Geometry: final body of the model. Coordinates: model frame, mm. A direction names the side the tool comes from. Round coordinates to 2 decimals unless told otherwise and drop trailing zeros. Loops run counter-clockwise (first coordinate to the right, second up) from the corner with the lowest first, then second, coordinate; pieces in that order, holes last. Notation, with made-up numbers: (3.5, 75.5) - (35.5, 75.5) arc R21 ccw to (35.5, 113.5) - close; hole circle Ø7 at (21.5, -1.5). An arc over 180 degrees is marked (long way). Use CSV: the item, a comma, the result in double quotes.
from build123d import *

# Parameters (mm, degrees)
SKETCH1_W            = 76.2
SKETCH1_H            = 76.2
BOSS_EXTRUDE1_DEPTH  = 1.5875
SKETCH3_W            = 6.35
SKETCH3_H            = 3.175
SKETCH3_W_2          = 3.175
SKETCH3_H_2          = 6.35
BOSS_EXTRUDE2_DEPTH  = 12.7
SKETCH4_W            = 6.35
SKETCH4_H            = 14.2875
BOSS_EXTRUDE3_DEPTH  = 7.62
SKETCH5_W            = 14.2875
SKETCH5_H            = 6.35
BOSS_EXTRUDE4_DEPTH  = 7.62
SKETCH6_W            = 14.2875
SKETCH6_H            = 6.35
BOSS_EXTRUDE5_DEPTH  = 7.62
SKETCH7_R            = 1.984375
CUT_EXTRUDE2_DEPTH   = 67.217591743
BOSS_EXTRUDE6_DEPTH  = 76.2
CUT_EXTRUDE3_REACH   = 89.333
SKETCH9_W            = 63.5
SKETCH9_H            = 12.7
BOSS_EXTRUDE7_DEPTH  = 6.35
BOSS_EXTRUDE8_DEPTH  = 6.35
SKETCH12_W           = 7.62
SKETCH12_H           = 12.7
SKETCH12_R           = 1.984375
CUT_EXTRUDE4_DEPTH   = 30.48
SKETCH13_W           = 6.35
SKETCH13_H           = 7.62
CUT_EXTRUDE5_DEPTH   = 30.48
SKETCH15_W           = 6.35
SKETCH15_H           = 12.7
CUT_EXTRUDE6_DEPTH   = 30.48
BOSS_EXTRUDE9_DEPTH  = 14.2875
SKETCH17_R           = 2.5
CUT_EXTRUDE7_DEPTH   = 24.9555
SKETCH18_R           = 2.5
CUT_EXTRUDE8_DEPTH   = 11.43
BOSS_EXTRUDE10_DEPTH = 3.556
SKETCH20_W           = 16
SKETCH20_H           = 16
SKETCH20_R           = 2.5
BOSS_EXTRUDE11_DEPTH = 14.2875
SKETCH21_R           = 2.5
CUT_EXTRUDE9_DEPTH   = 31.0515
SKETCH22_R           = 2.5
CUT_EXTRUDE10_DEPTH  = 10.16
SKETCH23_W           = 23.556
SKETCH23_H           = 14.2875
BOSS_EXTRUDE12_DEPTH = 1.27
SKETCH24_W           = 6.35
SKETCH24_H           = 7.62
CUT_EXTRUDE11_DEPTH  = 30.988
SKETCH25_W           = 7.62
SKETCH25_H           = 12.7
CUT_EXTRUDE12_DEPTH  = 30.988
SKETCH26_W           = 12.7
SKETCH26_H           = 12.7
BOSS_EXTRUDE13_DEPTH = 12.192
SKETCH28_W           = 12.7
SKETCH28_H           = 12.7
BOSS_EXTRUDE15_DEPTH = 12.2555
SKETCH29_W           = 12.7
SKETCH29_H           = 12.367297847
BOSS_EXTRUDE16_DEPTH = 8.9535
SKETCH30_W           = 6.317197846
SKETCH30_H           = 6.27
CUT_EXTRUDE13_DEPTH  = 32.8295
SKETCH27_W           = 10
SKETCH27_H           = 10
BOSS_EXTRUDE17_DEPTH = 14.2875


with BuildPart() as part:
    # Sketch1 → Boss-Extrude1 (new body)
    with BuildSketch(Plane.XY):
        Rectangle(SKETCH1_W, SKETCH1_H)
    extrude(amount=BOSS_EXTRUDE1_DEPTH)

    # Sketch3 → Boss-Extrude2 (add)
    with BuildSketch(Plane.XY.offset(1.5875)):
        with Locations((-34.925, 36.5125)):
            Rectangle(SKETCH3_W, SKETCH3_H)
        with Locations((34.925, 36.5125)):
            Rectangle(SKETCH3_W, SKETCH3_H)
        with Locations((-36.5125, -34.925)):
            Rectangle(SKETCH3_W_2, SKETCH3_H_2)
        with Locations((36.5125, -34.925)):
            Rectangle(SKETCH3_W_2, SKETCH3_H_2)
    extrude(amount=BOSS_EXTRUDE2_DEPTH)

    # Sketch4 → Boss-Extrude3 (add)
    with BuildSketch(Plane(origin=(0, 38.1, 0), x_dir=(1, 0, 0), z_dir=(0, 1, 0))):
        with Locations((-34.925, -7.14375)):
            Rectangle(SKETCH4_W, SKETCH4_H)
        with Locations((34.925, -7.14375)):
            Rectangle(SKETCH4_W, SKETCH4_H)
    extrude(amount=BOSS_EXTRUDE3_DEPTH)

    # Sketch5 → Boss-Extrude4 (add)
    with BuildSketch(Plane(origin=(38.1, 0, 0), x_dir=(0, 0, -1), z_dir=(1, 0, 0))):
        with Locations((-7.14375, -34.925)):
            Rectangle(SKETCH5_W, SKETCH5_H)
    extrude(amount=BOSS_EXTRUDE4_DEPTH)

    # Sketch6 → Boss-Extrude5 (add)
    with BuildSketch(Plane.ZY.offset(38.1)):
        with Locations((7.14375, -34.925)):
            Rectangle(SKETCH6_W, SKETCH6_H)
    extrude(amount=BOSS_EXTRUDE5_DEPTH)

    # Sketch7 → Cut-Extrude2 (cut, through all)
    with BuildSketch(Plane(origin=(0, 0, 0), x_dir=(-1, 0, 0), z_dir=(0, 0, -1))):
        with Locations((-34.925, 41.39168957)):
            Circle(SKETCH7_R)
        with Locations((34.925, 41.39168957)):
            Circle(SKETCH7_R)
        with Locations((-41.275, -34.925)):
            Circle(SKETCH7_R)
        with Locations((41.275, -34.925)):
            Circle(SKETCH7_R)
    extrude(amount=-CUT_EXTRUDE2_DEPTH, mode=Mode.SUBTRACT)

    # Sketch8 → Boss-Extrude6 (add)
    with BuildSketch(Plane.ZY.offset(38.1)):
        Polygon((1.5875, 25.732702153), (14.2875, 34.925), (1.5875, 34.925), align=None)
    extrude(amount=-BOSS_EXTRUDE6_DEPTH)

    # Sketch9 → Cut-Extrude3 (cut, up to next)
    with BuildSketch(Plane(origin=(0, 34.925, 0), x_dir=(1, 0, 0), z_dir=(0, 1, 0)), mode=Mode.PRIVATE) as cut_extrude3_sk1:
        with Locations((0, -7.9375)):
            Rectangle(SKETCH9_W, SKETCH9_H)
    cut_extrude3_tool1 = extrude(cut_extrude3_sk1.sketch, amount=-CUT_EXTRUDE3_REACH, mode=Mode.PRIVATE) & part.part
    add(cut_extrude3_tool1.solids().sort_by_distance((0, 34.925, 7.9375))[0], mode=Mode.SUBTRACT)

    # Sketch10 → Boss-Extrude7 (add)
    with BuildSketch(Plane.XZ.offset(38.1)):
        Polygon((-26.257396371, 1.5875), (-34.925, 14.2875), (-34.925, 1.5875), align=None)
        Polygon((34.925, 14.2875), (26.257396371, 1.5875), (34.925, 1.5875), align=None)
    extrude(amount=-BOSS_EXTRUDE7_DEPTH)

    # Sketch11 → Boss-Extrude8 (add)
    with BuildSketch(Plane.XZ.offset(38.1)):
        Polygon((-45.72, 14.2875), (-45.72, 0), (45.72, 0), (45.72, 14.2875), (34.925, 14.2875), (26.257396371, 1.5875), (-26.257396371, 1.5875), (-34.925, 14.2875), align=None)
    extrude(amount=BOSS_EXTRUDE8_DEPTH)

    # Sketch12 → Cut-Extrude4 (cut)
    with BuildSketch(Plane(origin=(0, 0, 0), x_dir=(-1, 0, 0), z_dir=(0, 0, -1))):
        with Locations((-41.91, -38.1)):
            Rectangle(SKETCH12_W, SKETCH12_H)
        with Locations((-41.275, -34.925)):
            Circle(SKETCH12_R, mode=Mode.SUBTRACT)
    extrude(amount=-CUT_EXTRUDE4_DEPTH, mode=Mode.SUBTRACT)

    # Sketch13 → Cut-Extrude5 (cut)
    with BuildSketch(Plane(origin=(0, 0, 0), x_dir=(-1, 0, 0), z_dir=(0, 0, -1))):
        with Locations((-34.925, 41.91)):
            Rectangle(SKETCH13_W, SKETCH13_H)
    extrude(amount=-CUT_EXTRUDE5_DEPTH, mode=Mode.SUBTRACT)

    # Sketch15 → Cut-Extrude6 (cut)
    with BuildSketch(Plane(origin=(0, 38.1, 0), x_dir=(1, 0, 0), z_dir=(0, 1, 0))):
        with Locations((34.925, -7.9375)):
            Rectangle(SKETCH15_W, SKETCH15_H)
    extrude(amount=-CUT_EXTRUDE6_DEPTH, mode=Mode.SUBTRACT)

    # Sketch16 → Boss-Extrude9 (add)
    with BuildSketch(Plane(origin=(0, 0, 0), x_dir=(-1, 0, 0), z_dir=(0, 0, -1))):
        Polygon((-38.1, 38.1), (-38.1, 43.1), (-18.1, 43.1), (-18.1, 29.1), (-38.1, 29.1), align=None)
    extrude(amount=-BOSS_EXTRUDE9_DEPTH)

    # Sketch17 → Cut-Extrude7 (cut)
    with BuildSketch(Plane(origin=(0, 0, 0), x_dir=(-1, 0, 0), z_dir=(0, 0, -1))):
        with Locations((-23.1, 38.1)):
            Circle(SKETCH17_R)
    extrude(amount=-CUT_EXTRUDE7_DEPTH, mode=Mode.SUBTRACT)

    # Sketch18 → Cut-Extrude8 (cut)
    with BuildSketch(Plane(origin=(0, 0, 0), x_dir=(-1, 0, 0), z_dir=(0, 0, -1))):
        Polygon((-25.409401077, 34.1), (-20.790598923, 34.1), (-18.481197846, 38.1), (-20.790598923, 42.1), (-25.409401077, 42.1), (-27.718802154, 38.1), align=None)
        with Locations((-23.1, 38.1)):
            Circle(SKETCH18_R, mode=Mode.SUBTRACT)
    extrude(amount=-CUT_EXTRUDE8_DEPTH, mode=Mode.SUBTRACT)

    # Sketch19 → Boss-Extrude10 (add)
    with BuildSketch(Plane.ZY.offset(-18.1)):
        Polygon((1.5875, 29.1), (14.2875, 29.1), (14.2875, 43.1), (0, 43.1), (0, 38.1), (1.5875, 38.1), align=None)
    extrude(amount=BOSS_EXTRUDE10_DEPTH)

    # Sketch20 → Boss-Extrude11 (add)
    with BuildSketch(Plane(origin=(0, 0, 0), x_dir=(-1, 0, 0), z_dir=(0, 0, -1))):
        with Locations((-23.1, -5.9)):
            Rectangle(SKETCH20_W, SKETCH20_H)
        with Locations((-23.1, -5.9)):
            Circle(SKETCH20_R, mode=Mode.SUBTRACT)
    extrude(amount=-BOSS_EXTRUDE11_DEPTH)

    # Sketch21 → Cut-Extrude9 (cut)
    with BuildSketch(Plane(origin=(0, 0, 0), x_dir=(-1, 0, 0), z_dir=(0, 0, -1))):
        with Locations((-23.1, -5.9)):
            Circle(SKETCH21_R)
    extrude(amount=-CUT_EXTRUDE9_DEPTH, mode=Mode.SUBTRACT)

    # Sketch22 → Cut-Extrude10 (cut)
    with BuildSketch(Plane(origin=(0, 0, 0), x_dir=(-1, 0, 0), z_dir=(0, 0, -1))):
        Polygon((-25.409401077, -9.9), (-20.790598923, -9.9), (-18.481197846, -5.9), (-20.790598923, -1.9), (-25.409401077, -1.9), (-27.718802154, -5.9), align=None)
        with Locations((-23.1, -5.9)):
            Circle(SKETCH22_R, mode=Mode.SUBTRACT)
    extrude(amount=-CUT_EXTRUDE10_DEPTH, mode=Mode.SUBTRACT)

    # Sketch23 → Boss-Extrude12 (add)
    with BuildSketch(Plane(origin=(0, 43.1, 0), x_dir=(1, 0, 0), z_dir=(0, 1, 0))):
        with Locations((26.322, -7.14375)):
            Rectangle(SKETCH23_W, SKETCH23_H)
    extrude(amount=BOSS_EXTRUDE12_DEPTH)

    # Sketch24 → Cut-Extrude11 (cut)
    with BuildSketch(Plane(origin=(0, 0, 0), x_dir=(-1, 0, 0), z_dir=(0, 0, -1))):
        with Locations((34.925, 41.91)):
            Rectangle(SKETCH24_W, SKETCH24_H)
    extrude(amount=-CUT_EXTRUDE11_DEPTH, mode=Mode.SUBTRACT)

    # Sketch25 → Cut-Extrude12 (cut)
    with BuildSketch(Plane(origin=(0, 0, 0), x_dir=(-1, 0, 0), z_dir=(0, 0, -1))):
        with Locations((41.91, -38.1)):
            Rectangle(SKETCH25_W, SKETCH25_H)
    extrude(amount=-CUT_EXTRUDE12_DEPTH, mode=Mode.SUBTRACT)

    # Sketch26 → Boss-Extrude13 (add)
    with BuildSketch(Plane(origin=(38.1, 0, 0), x_dir=(0, 0, -1), z_dir=(1, 0, 0))):
        with Locations((-7.9375, -38.1)):
            Rectangle(SKETCH26_W, SKETCH26_H)
    extrude(amount=-BOSS_EXTRUDE13_DEPTH)

    # Sketch28 → Boss-Extrude15 (add)
    with BuildSketch(Plane.ZY.offset(38.1)):
        with Locations((7.9375, -38.1)):
            Rectangle(SKETCH28_W, SKETCH28_H)
    extrude(amount=-BOSS_EXTRUDE15_DEPTH)

    # Sketch29 → Boss-Extrude16 (add)
    with BuildSketch(Plane.ZY.offset(38.1)):
        with Locations((7.9375, 31.916351076)):
            Rectangle(SKETCH29_W, SKETCH29_H)
    extrude(amount=-BOSS_EXTRUDE16_DEPTH)

    # Sketch30 → Cut-Extrude13 (cut)
    with BuildSketch(Plane(origin=(0, 0, 0), x_dir=(-1, 0, 0), z_dir=(0, 0, -1))):
        with Locations((-34.941401077, 41.235)):
            Rectangle(SKETCH30_W, SKETCH30_H)
    extrude(amount=-CUT_EXTRUDE13_DEPTH, mode=Mode.SUBTRACT)

    # Sketch27 → Boss-Extrude17 (add)
    with BuildSketch(Plane(origin=(0, 0, 0), x_dir=(-1, 0, 0), z_dir=(0, 0, -1))):
        with Locations((20.007888644, -3.175)):
            Rectangle(SKETCH27_W, SKETCH27_H)
    extrude(amount=-BOSS_EXTRUDE17_DEPTH)


solid = part.part
Item 1: Mould query, pull axis X, two halves, no side actions, for faces 1 (the flat face through (19.652, 36.072, 5.635)), 2 (the flat face through (-20, -8.175, 8)), 3 (the flat face through (-25.008, -3, 8)). Classes: released by +X, released by -X, zero draft, split by the parting line, or undercut.
Final values:
face 1,"undercut"
face 2,"zero draft"
face 3,"released by -X"
Item 2: Reachability of faces 4 (the flat face through (19.62, -3.93, 5.01)), 5 (the flat face through (31.1, -6, 8)), 6 (the flat face through (-24, 38.1, 1)) from +Z, -Z, +X, -X, +Y, -Y: full face, straight path, thin tool, end or side. Return the list, or none.
Final values:
face 4,"-Z"
face 5,"+Z, +X"
face 6,"+Z, -Z, -X, +Y"
Item 3: Section C-C on x = -6. Return the cut outline in (y, z), plus the area to 3 significant figures.
Final values:
outline,"(-44.45, 0) - (38.1, 0) - (38.1, 1.59) - (-44.45, 1.59) - close"
area,"131 mm²"
Item 4: Section D-D on y = -33. Return the cut outline in (x, z).
Final values:
outline,"(-38.1, 0) - (38.1, 0) - (38.1, 14.29) - (25.91, 14.29) - (25.91, 1.59) - (-25.84, 1.59) - (-25.84, 14.29) - (-38.1, 14.29) - close"
Item 5: Material intervals for line 1 (Y direction, x = 23.1, z = 12.1); line 2 (X direction, y = -33.5, z = 10.75); line 3 (Z direction, x = 12, y = 18.5), sorted ascending.
Final values:
line 1,"y = -13.9 to -8.4, -3.4 to 2.1, 29.1 to 35.6, 40.6 to 44.37"
line 2,"x = -38.1 to -25.84, 25.91 to 38.1"
line 3,"z = 0 to 1.59"
Item 6: Pin query (flat end, axial travel): P1, Ø3, axis at y = -3, z = 6, coming from the -X side; P2, Ø6.5, axis at x = 23.5, y = 38, coming from the -Z side; P3, Ø1.9, axis at x = 35.5, z = 4.5, coming from the +Y side. Return the tip coordinate at first contact, or that it passes through.
Final values:
P1,"stops at x = -25.01"
P2,"stops at z = 11.43"
P3,"stops at y = 38.1"
Item 7: Section B-B on y = 0. Return the cut outline in (x, z), plus the area to 3 significant figures.
Final values:
outline,"(-38.1, 0) - (38.1, 0) - (38.1, 1.59) - (31.1, 1.59) - (31.1, 14.29) - (15.1, 14.29) - (15.1, 1.59) - (-15.01, 1.59) - (-15.01, 14.29) - (-25.01, 14.29) - (-25.01, 1.59) - (-38.1, 1.59) - close"
area,"451 mm²"
Item 8: Section A-A on z = 5.75. Give the number of separate pieces and of enclosed holes in the cut face, plus the area to 3 significant figures.
Final values:
separate pieces,"6"
enclosed holes,"2"
area,"986 mm²"
